Check sheet for the modelled part. Datum: model origin and axes. Units: mm. Face numbers are marked on the shaded views. A direction names the side the tool comes from. Round coordinates to 2 decimals unless told otherwise and drop trailing zeros. Loops run counter-clockwise (first coordinate to the right, second up) from the corner with the lowest first, then second, coordinate; pieces in that order, holes last. Notation, with made-up numbers: (14.5, 24.5) -> (34.5, 24.5) arc R19 ccw to (34.5, 29.5) -> close; hole circle Ø1 at (61.5, 28). An arc over 180 degrees is marked (long way). One line per item, written item: value. Start each with the question number.
1. Cross-section at D-D on y = -8. Record the cut outline in (x, z).
2. Cross-section at C-C on z = -0.75. Record the cut outline in (x, y), then the cut area to 3 significant figures.
3. Cross-section at B-B on x = 12.2. Record the cut outline in (y, z), then the cut area to 3 significant figures.
4. Material ranges on L1, parallel to Y at x = 12.2, z = -0.7; L2, parallel to X at y = -2.75, z = -1.75; L3, parallel to X at y = 9, z = -0.5, recorded low to high.
5. Go/stop test with flat-tipped pins: pin 1 (1.5 mm diameter, centred on y = 5, z = 0.5, fed in from -X); pin 2 (1.5 mm diameter, centred on x = -2.5, z = -1.5, fed in from +Y); pin 3 (2 mm diameter, centred on x = 2, z = 2.5, fed in from +Y); pin 4 (12.5 mm diameter, centred on x = 12.2, y = 0.75, fed in from -Z). Record where each tip stops, or that it passes through.
6. Set-up check for the marked faces 4, 5 and 6: record each of +Z, -Z, +X, -X, +Y, -Y from which the full face is reachable in a straight line by a thin tool's end or side.
7. Release check for a two-part mould opening along X. For the marked faces 1, 2 and 3 record: +X half, -X half, draft (parallel to the pull), parting line (faces both ways), or undercut.
8. Cross-section at A-A on y = 0.75. Record the cut outline in (x, z), then the cut area to 3 significant figures.
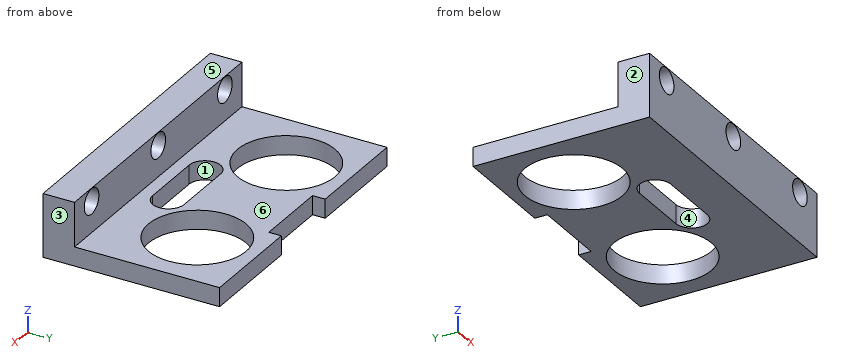
Autodesk Inventor part; units mm, degrees
ref_plane "YZ Plane" through (0, 0, 0) normal (1, 0, 0) x (0, 1, 0)
ref_plane "XZ Plane" through (0, 0, 0) normal (0, 1, 0) x (-1, 0, 0)
ref_plane "XY Plane" through (0, 0, 0) normal (0, 0, 1) x (1, 0, 0)
sketch "Эскиз3" plane through (0, 0, 0) normal (0, 0, 1) x (1, 0, 0)
  line L0 (22.95, -10.5) -> (22.95, 10.5)
  line L1 (-22.95, 10.5) -> (-22.95, -10.5)
  line L2 (-22.95, -10.5) -> (22.95, 10.5) construction
  line L3 (22.95, -10.5) -> (-22.95, 10.5) construction
  line L4 (-6, 10.5) -> (-22.95, 10.5) construction
  line L5 (6, 10.5) -> (22.95, 10.5) construction
  line L6 (22.95, 0) -> (19.95, 0) construction
  line L7 (16.3868, 10.5) -> (16.3868, 8.5) construction
  line L8 (17.599, 8.5) -> (14.8742, 8.5) construction
  line L9 (19.95, 1.7069) -> (19.95, -1.7382) construction
  line L10 (16.2366, -10.5) -> (16.2366, -7) construction
  line L11 (17.599, -7) -> (14.2766, -7) construction
  circle A0 centre (12.2, 0.75) radius 7.75
  line L12 (0, 10.5) -> (0, -10.5) construction
  line L13 (-22.95, 0) -> (-19.95, 0) construction
  line L14 (-16.3868, 10.5) -> (-16.3868, 8.5) construction
  line L15 (-17.599, 8.5) -> (-14.8742, 8.5) construction
  line L16 (-19.95, 1.7069) -> (-19.95, -1.7382) construction
  line L17 (-16.2366, -10.5) -> (-16.2366, -7) construction
  line L18 (-17.599, -7) -> (-14.2766, -7) construction
  circle A1 centre (-12.2, 0.75) radius 7.75
  line L19 (-22.95, 0) -> (22.95, 0) construction
  line L20 (0, 8.5) -> (0, -5.5) construction
  line L21 (0, -5.5) -> (5, -5.5)
  line L22 (0, -5.5) -> (-5, -5.5)
  line L23 (-5, -10.5) -> (5, -10.5)
  arc A2 (-5, -5.5) -> (-5, -10.5) centre (-5, -8) ccw
  arc A3 (5, -10.5) -> (5, -5.5) centre (5, -8) ccw
  line L24 (-22.95, -10.5) -> (-22.95, -12.5)
  line L25 (-22.95, -12.5) -> (22.95, -12.5)
  line L26 (22.95, -12.5) -> (22.95, -10.5)
  line L27 (0, 8.5) -> (6, 8.5)
  line L28 (0, 8.5) -> (-6, 8.5)
  line L29 (-6, 8.5) -> (-6, 10.5)
  line L30 (6, 8.5) -> (6, 10.5)
  line L31 (22.95, 10.5) -> (6, 10.5)
  line L32 (-6, 10.5) -> (-22.95, 10.5)
  point P0 (0, 0)
  point P1 (5, -5.5)
  point P2 (-5, -5.5)
  dimension "d23" = 45.9
  dimension "d24" = 21
  dimension "d26" = 3
  dimension "d27" = 2
  dimension "d29" = 3.5
  dimension "d30" = 16
  dimension "d31" = 5
  dimension "d32" = 2.5
  dimension "d35" = 2
  dimension "d47" = 6
  dimension "d48" = 6
extrude "Выдавливание5" add sketch "Эскиз3" against normal blind 3
sketch "Эскиз4" plane through (0, 0, 0) normal (0, 0, 1) x (1, 0, 0)
  line L0 (-22.95, -12.5) -> (22.95, -12.5)
  line L1 (22.95, -12.5) -> (22.95, -17.5)
  line L2 (22.95, -17.5) -> (-22.95, -17.5)
  line L3 (-22.95, -17.5) -> (-22.95, -12.5)
  line L4 (22.95, -12.5) -> (-22.95, -12.5)
  point P0 (0, 0)
  dimension "d36" = 5
extrude "Выдавливание6" add sketch "Эскиз4" along normal blind 7 and the other way blind 3
sketch "Эскиз6" plane through (-22.95, -12.5, 0) normal (0, 1, 0) x (1, 0, 0)
  line L0 (45.9, 0) -> (0, 0)
  line L1 (0, -7) -> (0, 0)
  line L2 (45.9, -7) -> (0, -7)
  line L3 (45.9, 0) -> (45.9, -7)
  line L4 (45.9, 0) -> (45.9, -7) construction
  line L5 (45.9, -3.5) -> (0, -3.5) construction
  line L6 (0, -7) -> (0, 0) construction
  line L7 (0, -7) -> (45.9, -7) construction
  line L8 (22.95, -7) -> (22.95, 0) construction
  circle A0 centre (41.2273, -4.9258) radius 2
  circle A1 centre (4.6727, -4.9258) radius 2
  line L9 (45.9, -4.1809) -> (0, -4.1809) construction
  circle A2 centre (22.95, -4.9258) radius 2
  dimension "d50" = 4
extrude "Выдавливание8" cut sketch "Эскиз6" against normal blind 10 contours A0 | A1 | A2
properties part number "Mount for US"
Taken from the geometry:
1. outline: (-22.95, -3) -> (-7.5, -3) -> (-7.5, 0) -> (-22.95, 0) -> close; (7.5, -3) -> (22.95, -3) -> (22.95, 0) -> (7.5, 0) -> close
2. outline: (-22.95, -17.5) -> (22.95, -17.5) -> (22.95, 10.5) -> (6, 10.5) -> (6, 8.5) -> (-6, 8.5) -> (-6, 10.5) -> (-22.95, 10.5) -> close; hole circle Ø15.5 at (-12.2, 0.75); hole (-5, -10.5) -> (5, -10.5) arc R2.5 ccw to (5, -5.5) -> (-5, -5.5) arc R2.5 ccw to start; hole circle Ø15.5 at (12.2, 0.75)
2. area: 814 mm2
3. outline: (-17.5, -3) -> (-7, -3) -> (-7, 0) -> (-12.5, 0) -> (-12.5, 7) -> (-17.5, 7) -> close; (8.5, -3) -> (10.5, -3) -> (10.5, 0) -> (8.5, 0) -> close
3. area: 72.5 mm2
4. L1: y = -17.5 to -7, 8.5 to 10.5
4. L2: x = -22.95 to -19.11, -5.29 to 5.29, 19.11 to 22.95
4. L3: x = -22.95 to -6, 6 to 22.95
5. pin 1: stops at x = -22.95
5. pin 2: stops at y = 8.5
5. pin 3: stops at y = -12.5
5. pin 4: passes through
6. face 4: +Z, -Z
6. face 5: +Z, +X, -X, +Y, -Y
6. face 6: +Z, +X, -X, +Y
7. face 1: undercut
7. face 2: -X half
7. face 3: +X half
8. outline: (-22.95, -3) -> (-19.95, -3) -> (-19.95, 0) -> (-22.95, 0) -> close; (-4.45, -3) -> (4.45, -3) -> (4.45, 0) -> (-4.45, 0) -> close; (19.95, -3) -> (22.95, -3) -> (22.95, 0) -> (19.95, 0) -> close
8. area: 44.7 mm2
